For this review, take the finished solid that the model builds, in its own axes (mm). A direction names the side the tool comes from. Coordinates: 2 decimals unless noted, no trailing zeros. Loops run counter-clockwise (first coordinate to the right, second up) from the corner with the lowest first, then second, coordinate; pieces in that order, holes last. Notation, with made-up numbers: (-14.5, -15) -> (35.5, -15) arc R33 cw to (35.5, 18) -> close; hole circle Ø8 at (16.5, -10). An arc over 180 degrees is marked (long way). Use a Markdown table: item, result.
Autodesk Inventor part; units mm, degrees
ref_plane "YZ Plane" through (0, 0, 0) normal (1, 0, 0) x (0, 1, 0)
ref_plane "XZ Plane" through (0, 0, 0) normal (0, 1, 0) x (-1, 0, 0)
ref_plane "XY Plane" through (0, 0, 0) normal (0, 0, 1) x (1, 0, 0)
sketch "Sketch1" plane through (0, 0, 0) normal (0, 0, 1) x (1, 0, 0)
  circle A0 centre (0, 0) radius 2.413
  dimension "d0" = 4.826
extrude "Extrusion1" add sketch "Sketch1" along normal blind 12.7
sketch "Sketch2" plane through (0, 0, 0) normal (0, 1, 0) x (-1, 0, 0)
  line L0 (0, 0) -> (0, -2.5654)
  line L1 (0, 0) -> (4.3239, 0)
  line L2 (0, -2.5654) -> (2.032, -2.5654)
  line L3 (4.3239, 0) -> (4.3239, 3.8864) construction
  arc A0 (4.5568, -0.3781) -> (4.3239, 0) centre (4.3239, -0.2608) ccw
  arc A1 (2.032, -2.5654) -> (4.5568, -0.3781) centre (0.6382, 1.5944) ccw
  line L4 (4.5847, 0.6553) -> (4.5847, -0.2608) construction
  dimension "d3" = 2.5654
  dimension "d6" = 2.032
  dimension "d12" = 4.5847
revolve "Revolution1" add sketch "Sketch2" angle 360 about axis through (0, 0, 0) along (0, 0, -1)
sketch "Sketch3" plane through (0, 0, -2.5654) normal (0, 0, -1) x (-1, 0, 0)
  circle A0 centre (0, 0) radius 2.032
  line L0 (-0.9165, 1.5875) -> (0.9165, 1.5875)
  line L1 (0.9165, 1.5875) -> (1.8331, 0)
  line L2 (1.8331, 0) -> (0.9165, -1.5875)
  line L3 (0.9165, -1.5875) -> (-0.9165, -1.5875)
  line L4 (-0.9165, -1.5875) -> (-1.8331, 0)
  line L5 (-1.8331, 0) -> (-0.9165, 1.5875)
  dimension "d8" = 3.175
extrude "Extrusion2" cut sketch "Sketch3" against normal blind 1.5875 contours L0 L1 L2 L3 L4 L5
chamfer "Chamfer1" distance 0.508 angle 45 1 edges at (-2.413, 0, 12.7)
thread "Thread1"
properties part number "10-32 x500 button head" material "Steel"
(1) For line 1 along Z through (x, y) = (0.25, 1.25); line 2 along Z through (x, y) = (-3.5, -0.75); line 3 along Y through (x, z) = (-1, 0.25), list the stretches that pass through material, from the lowest coordinate up.
Found:
| item | result |
|---|---|
| line 1 | z = -0.98 to 12.7 |
| line 2 | z = -1.66 to 0 |
| line 3 | y = -2.2 to 2.2 |
(2) For faces 4 (the face through (-2, -2, 0)), 5 (the face through (0, -1.588, -2)), list the 3-axis set-ups (+Z, -Z, +X, -X, +Y, -Y) from which the entire face can be reached by the end or side of a thin tool; tool diameter is ignored.
Found:
| item | result |
|---|---|
| face 4 | +Z |
| face 5 | -Z |
(3) Mouldability with a two-part tool opening along Y and no side actions: class faces 1 (the face through (0, 0, 12.7)), 2 (the face through (-1.37, 0.8, -1.78)), 3 (the face through (-1.915, 1.468, 6.011)) as pulls with the +Y half, pulls with the -Y half, needs draft (parallel to the pull), parting line crosses it, or undercut.
Found:
| item | result |
|---|---|
| face 1 | needs draft |
| face 2 | undercut |
| face 3 | parting line crosses it |
(4) For pin 1 Ø2 at (x, z) = (-2.5, 4) entering from -Y; pin 2 Ø1.3 at (x, z) = (0.5, -1.5) entering from -Y; pin 3 Ø4 at (x, z) = (0, 5) entering from +Y, all flat-tipped, find the tip position at first contact; note any pin that passes through.
Found:
| item | result |
|---|---|
| pin 1 | stops at y = -1.89 |
| pin 2 | stops at y = -4.26 |
| pin 3 | stops at y = 2.41 |
(5) Take a section at A-A on z = 7.5. Write out the cut boundary in (x, y).
Found:
| item | result |
|---|---|
| outline | circle Ø4.83 at (0, 0) |
